The listing builds one solid part. Answer for the finished solid, in the listing's coordinates (mm). Give positions to 0.01 mm unless a question says otherwise; leave off trailing zeros. Order: outer loops, then holes, each group sorted by start corner. A loop starts at its lowest first (then second) coordinate and runs counter-clockwise, first axis right, second up. Notation, with made-up numbers: (82, 31.25) - (88, 31.25) arc R13 cw to (88, 50.25) - close; hole circle Ø5 at (34.25, 43.5). An arc over 180 degrees is marked (long way). Use a Markdown table: item, result. Add a question column.
1) Find section B-B, the plane y = 2. Determine the outline of the cut face in (x, z).
2) Find section C-C, the plane x = 2.25. Determine the outline of the cut face in (y, z).
3) Straight lines are drawn through the part: line 1 (Y direction, x = 0, z = 1.2); line 2 (Y direction, x = 3.25, z = -2); line 3 (X direction, y = -0.5, z = 0.6). For each, find the intervals that lie inside material, in ascending order.
4) Find section A-A, the plane x = 0. Determine the outline of the cut face in (y, z), plus the area to 3 significant figures.
5) The mould has two halves that part along X. Classify faces 1 (the face through (-2.15, 0.09, 0.04)), 2 (the face through (-2, -2, -2.5)): released by +X, released by -X, zero draft, split by the parting line, or undercut.
from build123d import *

# Parameters (mm, degrees)
BODYS_R                = 4
BODY_DEPTH             = 2.5
ENGAGEMENTCUT_DEPTH    = 7.184658438
ECCP_COUNT             = 20
MAJORDIAMETERCUTS_R    = 2.15
MAJORDIAMETERCUT_DEPTH = 8.537904218


with BuildPart() as part:
    # BodyS → Body (new, symmetric)
    with BuildSketch(Plane(origin=(0, 0, 0), x_dir=(-1, 0, 0), z_dir=(0, 0, -1))):
        Circle(BODYS_R)
    extrude(amount=BODY_DEPTH, both=True)

    # EngagementCutS → EngagementCut (cut, symmetric)
    with BuildSketch(Plane(origin=(0, 0, 0), x_dir=(-1, 0, 0), z_dir=(0, 0, -1))):
        with BuildLine():
            Line((0.3, 3.988734135), (0.15, 3.79703832))
            ThreePointArc((0.15, 3.79703832), (0, 3.8), (-0.15, 3.79703832))
            Line((-0.15, 3.79703832), (-0.3, 3.988734135))
            ThreePointArc((-0.3, 3.988734135), (0, 4), (0.3, 3.988734135))
        make_face()
    engagementcut = extrude(amount=ENGAGEMENTCUT_DEPTH, both=True, mode=Mode.SUBTRACT)

    # ECCP: EngagementCut ×20 about axis
    eccp_axis = Axis((0, 0, 0), (0, 0, 1))
    for i in range(1, ECCP_COUNT):
        add(engagementcut.rotate(eccp_axis, i * 360 / ECCP_COUNT), mode=Mode.SUBTRACT)

    # MajorDiameterCutS → MajorDiameterCut (cut, through all)
    with BuildSketch(Plane.XY.offset(2.5)):
        Circle(MAJORDIAMETERCUTS_R)
    extrude(amount=-MAJORDIAMETERCUT_DEPTH, mode=Mode.SUBTRACT)


solid = part.part
The answers:
| question | item | result |
|---|---|---|
| 1 | outline | (-3.46, -2.5) - (-0.79, -2.5) - (-0.79, 2.5) - (-3.46, 2.5) - close; (0.79, -2.5) - (3.46, -2.5) - (3.46, 2.5) - (0.79, 2.5) - close |
| 2 | outline | (-3.06, -2.5) - (3.06, -2.5) - (3.06, 2.5) - (-3.06, 2.5) - close |
| 3 | line 1 | -3.8 to -2.15, 2.15 to 3.8 |
| 3 | line 2 | -2.11 to 2.11 |
| 3 | line 3 | -3.97 to -2.09, 2.09 to 3.97 |
| 4 | outline | (-3.8, -2.5) - (-2.15, -2.5) - (-2.15, 2.5) - (-3.8, 2.5) - close; (2.15, -2.5) - (3.8, -2.5) - (3.8, 2.5) - (2.15, 2.5) - close |
| 4 | area | 16.5 mm2 |
| 5 | face 1 | undercut |
| 5 | face 2 | zero draft |
